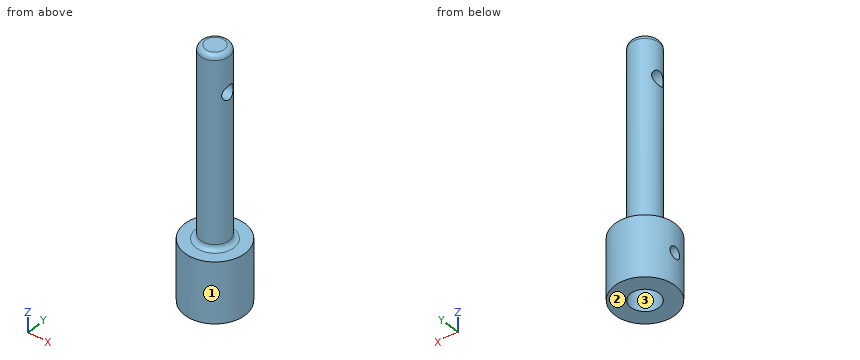
from build123d import *

# Parameters (mm, degrees)
SKETCH1_R               = 6.35
SKETCH1_R_2             = 3
BOSS_EXTRUDE1_DEPTH     = 11
SKETCH2_R               = 6.35
BOSS_EXTRUDE2_DEPTH     = 2
SKETCH3_R               = 3
BOSS_EXTRUDE3_DEPTH     = 40
CUT_EXTRUDE1_DEPTH      = 4
CUT_EXTRUDE1_DEPTH_BACK = 30
SKETCH4_R               = 1.25
FILLET1_R               = 1
FILLET2_R               = 1
CUT_EXTRUDE2_DEPTH      = 54.755418355
CUT_EXTRUDE2_DEPTH_BACK = 54.755418355
SKETCH5_R               = 1.5
SKETCH6_R               = 6.35
CUT_EXTRUDE3_DEPTH      = 0.2


with BuildPart() as part:
    # Sketch1 → Boss-Extrude1 (new body)
    with BuildSketch(Plane.XY):
        Circle(SKETCH1_R)
        Circle(SKETCH1_R_2, mode=Mode.SUBTRACT)
    extrude(amount=BOSS_EXTRUDE1_DEPTH)

    # Sketch2 → Boss-Extrude2 (add)
    with BuildSketch(Plane.XY.offset(11)):
        Circle(SKETCH2_R)
    extrude(amount=BOSS_EXTRUDE2_DEPTH)

    # Sketch3 → Boss-Extrude3 (add)
    with BuildSketch(Plane.XY.offset(13)):
        Circle(SKETCH3_R)
    extrude(amount=BOSS_EXTRUDE3_DEPTH)

    # Sketch4 → Cut-Extrude1 (cut, two sides: drawn at the far end of the back side and taken through both)
    with BuildSketch(Plane(origin=(0, 0, 0), x_dir=(0, 0, -1), z_dir=(1, 0, 0)).offset(-CUT_EXTRUDE1_DEPTH_BACK)):
        with Locations((-7, 0)):
            Circle(SKETCH4_R)
    extrude(amount=CUT_EXTRUDE1_DEPTH + CUT_EXTRUDE1_DEPTH_BACK, mode=Mode.SUBTRACT)

    # Fillet1
    fillet1_edges = [part.edges().sort_by_distance(p)[0] for p in [
        (-3, 0, 13),
    ]]
    fillet(fillet1_edges, radius=FILLET1_R)

    # Fillet2
    fillet2_edges = [part.edges().sort_by_distance(p)[0] for p in [
        (-3, 0, 53),
    ]]
    fillet(fillet2_edges, radius=FILLET2_R)

    # Sketch5 → Cut-Extrude2 (cut, two sides: drawn at the far end of the back side and taken through both)
    with BuildSketch(Plane(origin=(0, 0, 0), x_dir=(0, 0, -1), z_dir=(1, 0, 0)).offset(-CUT_EXTRUDE2_DEPTH_BACK)):
        with Locations(Location((-44.6, 0, 0), (0, 0, 179.999999999))):
            Circle(SKETCH5_R)
    extrude(amount=CUT_EXTRUDE2_DEPTH + CUT_EXTRUDE2_DEPTH_BACK, mode=Mode.SUBTRACT)

    # Sketch6 → Cut-Extrude3 (cut)
    with BuildSketch(Plane(origin=(0, 0, 0), x_dir=(-1, 0, 0), z_dir=(0, 0, -1))):
        Circle(SKETCH6_R)
    extrude(amount=-CUT_EXTRUDE3_DEPTH, mode=Mode.SUBTRACT)


solid = part.part
Geometry: final body of the model. Coordinates: model frame, mm. Face numbers are marked on the shaded views. Coordinates: 2 decimals unless noted, no trailing zeros. Loops run counter-clockwise (first coordinate to the right, second up) from the corner with the lowest first, then second, coordinate; pieces in that order, holes last. Notation, with made-up numbers: M -8.75,-40 L 34.25,-40 A16 cw 34.25,-26 Z; hole C 37.5,83 d4. An arc over 180 degrees is marked long. One line per item, written item: value. Start each with the question number.
1) Cut plane A-A (y = 0). Return loops of the section in (x, z).
2) Draft query along X for the marked faces 1, 2 and 3. Return one class per face: released by +X, released by -X, zero draft, split by the parting line, or undercut.
3) Material intervals for L1, parallel to Z at x = -3.25, y = 2.75; L2, parallel to X at y = 0, z = 7.5; L3, parallel to Z at x = -1.25, y = -1.75, sorted ascending. Write a range as from..to.
4) Cut plane D-D (z = 44.6). Return loops of the section in (x, y), then the cut area to 3 significant figures.
5) Cut plane C-C (z = 28.5). Return loops of the section in (x, y), then the cut area to 3 significant figures.
6) Cut plane B-B (x = 0). Return loops of the section in (y, z), then the cut area to 3 significant figures.
7) Pin query (flat end, axial travel): P1, Ø2, axis at y = -3, z = 28, coming from the -X side; P2, Ø4, axis at x = 3, z = 43, coming from the -Y side; P3, Ø1.8, axis at x = 0.5, y = -0.5, coming from the -Z side. Return the tip coordinate at first contact, or that it passes through.
Evaluation:
1. outline: M -6.35,0.2 L -3,0.2 L -3,5.75 L -6.35,5.75 Z; M -6.35,8.25 L -3,8.25 L -3,11 L 3,11 L 3,8.25 L 4,8.25 L 4,5.75 L 3,5.75 L 3,0.2 L 6.35,0.2 L 6.35,13 L 4,13 A1 cw 3,14 L 3,43.1 L -3,43.1 L -3,14 A1 cw -4,13 L -6.35,13 Z; M -3,46.1 L 3,46.1 L 3,52 A1 ccw 2,53 L -2,53 A1 ccw -3,52 Z
2. face 1: split by the parting line
2. face 2: zero draft
2. face 3: undercut
3. L1: 0.2..13
3. L2: 4..6.35
3. L3: 11..52.99
4. outline: M -2.6,-1.5 A3 ccw 2.6,-1.5 Z; M -2.6,1.5 L 2.6,1.5 A3 ccw Z
4. area: 11.1 mm^2
5. outline: C 0,0 d6
5. area: 28.3 mm^2
6. outline: M -6.35,0.2 L -3,0.2 L -3,11 L 3,11 L 3,0.2 L 6.35,0.2 L 6.35,13 L 4,13 A1 cw 3,14 L 3,52 A1 ccw 2,53 L -2,53 A1 ccw -3,52 L -3,14 A1 cw -4,13 L -6.35,13 Z; hole C 0,44.6 d3
6. area: 331 mm^2
7. P1: x = -2.24
7. P2: y = -2.83
7. P3: z = 11
